Read the model definition and answer for the solid it produces. Units are mm, in the model's axes. A direction names the side the tool comes from. Coordinates: 2 decimals unless noted, no trailing zeros. Order: outer loops, then holes, each group sorted by start corner. A loop starts at its lowest first (then second) coordinate and runs counter-clockwise, first axis right, second up. Notation, with made-up numbers: (45.5, 52) - (82.5, 52) arc R29 ccw to (82.5, 86) - close; hole circle Ø3 at (-28, -34). An arc over 180 degrees is marked (long way). Use one line per item in the form item = value. Start each with the question number.
from build123d import *

# Parameters (mm, degrees)
MODEL_R             = 2
MODEL_R_2           = 3.05
MODEL_R_3           = 6.75
BOSS_EXTRUDE1_DEPTH = 10
SKETCH2_R           = 16.1
CUT_EXTRUDE1_DEPTH  = 10


with BuildPart() as part:
    # Model → Boss-Extrude1 (new body)
    with BuildSketch(Plane.XY):
        with BuildLine():
            Line((106.910569106, -1), (106.910569106, 3))
            ThreePointArc((106.910569106, 3), (106.031889449, 5.121320344), (103.910569106, 6))
            Line((103.910569106, 6), (75.910569106, 6))
            ThreePointArc((75.910569106, 6), (73.082141981, 4.828427125), (71.910569106, 2))
            Line((71.910569106, 2), (71.910569106, -3.03491552))
            ThreePointArc((71.910569106, -3.03491552), (70.73899623, -5.863342645), (67.910569106, -7.034915521))
            Line((67.910569106, -7.034915521), (31.910569106, -7.034915521))
            ThreePointArc((31.910569106, -7.034915521), (24.839501294, -4.105983332), (21.910569106, 2.96508448))
            Line((21.910569106, 2.96508448), (21.910569106, 50))
            ThreePointArc((21.910569106, 50), (24.839501294, 57.071067812), (31.910569106, 60))
            Line((31.910569106, 60), (61.910569106, 60))
            ThreePointArc((61.910569106, 60), (68.981636918, 57.071067812), (71.910569106, 50))
            Line((71.910569106, 50), (71.910569106, 40))
            ThreePointArc((71.910569106, 40), (74.839501294, 32.928932188), (81.910569106, 30))
            Line((81.910569106, 30), (96.910569106, 30))
            ThreePointArc((96.910569106, 30), (103.981636918, 32.928932188), (106.910569106, 40))
            Line((106.910569106, 40), (106.910569106, 50))
            ThreePointArc((106.910569106, 50), (109.839501294, 57.071067812), (116.910569106, 60))
            Line((116.910569106, 60), (146.910569106, 60))
            ThreePointArc((146.910569106, 60), (153.981636918, 57.071067812), (156.910569106, 50))
            Line((156.910569106, 50), (156.910569106, 5))
            ThreePointArc((156.910569106, 5), (153.981636918, -2.071067812), (146.910569106, -5))
            Line((146.910569106, -5), (110.910569106, -5))
            ThreePointArc((110.910569106, -5), (108.082141981, -3.828427125), (106.910569106, -1))
        make_face()
        with Locations((66.910569106, 18)):
            Circle(MODEL_R, mode=Mode.SUBTRACT)
        with Locations((46.910569106, 18)):
            Circle(MODEL_R_2, mode=Mode.SUBTRACT)
        with Locations((116.910569106, 10)):
            Circle(MODEL_R, mode=Mode.SUBTRACT)
        with Locations((146.910569106, 10)):
            Circle(MODEL_R, mode=Mode.SUBTRACT)
        with Locations((146.910569106, 50)):
            Circle(MODEL_R, mode=Mode.SUBTRACT)
        with Locations((116.910569106, 50)):
            Circle(MODEL_R, mode=Mode.SUBTRACT)
        with Locations((131.910569106, 30)):
            Circle(MODEL_R_3, mode=Mode.SUBTRACT)
        with Locations((86.910569106, 18)):
            Circle(MODEL_R_2, mode=Mode.SUBTRACT)
    extrude(amount=BOSS_EXTRUDE1_DEPTH)

    # Sketch2 → Cut-Extrude1 (cut)
    with BuildSketch(Plane.XY.offset(10)):
        with Locations((131.910569106, 30)):
            Circle(SKETCH2_R)
    extrude(amount=-CUT_EXTRUDE1_DEPTH, mode=Mode.SUBTRACT)


solid = part.part
Q1. For a pull along X with two mould halves and no side action, classify faces 1 (the cylindrical face through (24.918, -4.183, 4.93)), 2 (the flat face through (156.911, 28, 5)), 3 (the cylindrical face through (145.323, 48.783, 4.93)) as +X half, -X half, draft (parallel to the pull), parting line (faces both ways), or undercut.
Q2. Consider probe 1 along Y at (x, z) = (146, 2.25); probe 2 along X at (y, z) = (31, 4); probe 3 along X at (y, z) = (49, 7). Determine where each line is inside the solid, lowest interval first.
Q3. A cutting plane is placed at B-B (y = 10). Give the vertices of the cut face in (x, z).
Q4. A cutting plane is placed at A-A (z = 6.5). Give the number of separate pieces and of enclosed holes in the cut face, then the cut area to 3 significant figures.
Q5. A cutting plane is placed at C-C (x = 134.5). Give the vertices of the cut face in (y, z).
Q6. Given P1, Ø10, axis at x = 86.91, y = 18, coming from the +Z side; P2, Ø2, axis at y = 1.5, z = 4, coming from the -X side; P3, Ø2.5, axis at y = 0, z = 2.5, coming from the +X side; P4, Ø5, axis at x = 95.5, z = 2.5, coming from the +Y side, each flat-ended and moving along its own axis, determine where each tip first touches the part or whether it passes through.
Q7. A cutting plane is placed at D-D (y = 53.5). Give the vertices of the cut face in (x, z).
Q8. Which of the six approach directions +Z, -Z, +X, -X, +Y, -Y give full straight-line access (tool end or side, diameter ignored) to faces 4 (the flat face through (50, -7.035, 5)), 5 (the cylindrical face through (68.9, 57.15, 4.93)), 6 (the cylindrical face through (108.113, -3.859, 4.93))?
Result sheet:
q1.face_1 = -X half
q1.face_2 = +X half
q1.face_3 = undercut
q2.probe_1 = -5 to 8.22, 11.78 to 22.21, 37.79 to 48.22, 51.78 to 60
q2.probe_2 = 21.91 to 77.55, 101.27 to 115.84, 147.98 to 156.91
q2.probe_3 = 21.91 to 71.91, 106.91 to 115.18, 118.64 to 145.18, 148.64 to 156.91
q3.outline = (21.91, 0) - (114.91, 0) - (114.91, 10) - (21.91, 10) - close; (118.91, 0) - (144.91, 0) - (144.91, 10) - (118.91, 10) - close; (148.91, 0) - (156.91, 0) - (156.91, 10) - (148.91, 10) - close
q4.separate_pieces = 1
q4.enclosed_holes = 8
q4.area = 6,420 mm^2
q5.outline = (-5, 0) - (14.11, 0) - (14.11, 10) - (-5, 10) - close; (45.89, 0) - (60, 0) - (60, 10) - (45.89, 10) - close
q6.P1 = 10
q6.P2 = 21.92
q6.P3 = 156.18
q6.P4 = 30.06
q7.outline = (22.54, 0) - (71.28, 0) - (71.28, 10) - (22.54, 10) - close; (107.54, 0) - (156.28, 0) - (156.28, 10) - (107.54, 10) - close
q8.face_4 = +Z, -Z, +X, -X, -Y
q8.face_5 = +Z, -Z, +Y
q8.face_6 = +Z, -Z, -Y
